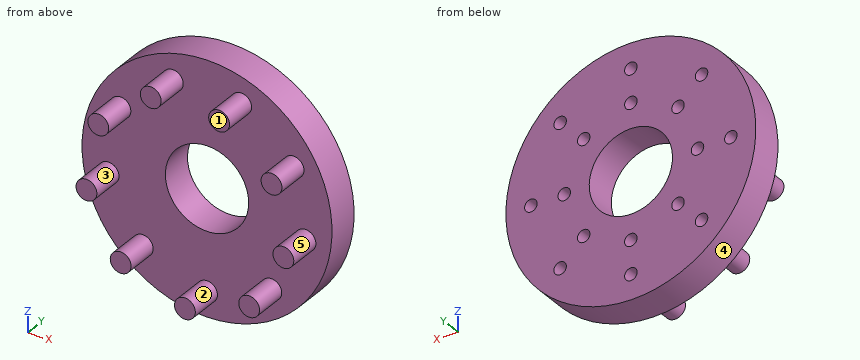
from build123d import *

# Parameters (mm, degrees)
SKETCH1_R           = 190.5
BOSS_EXTRUDE1_DEPTH = 50.8
SKETCH2_R           = 63.5
CUT_EXTRUDE1_DEPTH  = 275.155320941
SKETCH3_R           = 9.525
CUT_EXTRUDE2_DEPTH  = 42.926
SKETCH4_R           = 15.875
BOSS_EXTRUDE2_DEPTH = 50.8


with BuildPart() as part:
    # Sketch1 → Boss-Extrude1 (new body)
    with BuildSketch(Plane(origin=(0, 0, 0), x_dir=(1, 0, 0), z_dir=(0, 1, 0))):
        with Locations(Location((0, 0, 0), (0, 0, 270))):
            Circle(SKETCH1_R)
    extrude(amount=BOSS_EXTRUDE1_DEPTH)

    # Sketch2 → Cut-Extrude1 (cut, through all)
    with BuildSketch(Plane(origin=(0, 50.8, 0), x_dir=(1, 0, 0), z_dir=(0, 1, 0))):
        with Locations(Location((0, 0, 0), (0, 0, 270))):
            Circle(SKETCH2_R)
    extrude(amount=-CUT_EXTRUDE1_DEPTH, mode=Mode.SUBTRACT)

    # Sketch3 → Cut-Extrude2 (cut)
    with BuildSketch(Plane(origin=(0, 50.8, 0), x_dir=(1, 0, 0), z_dir=(0, 1, 0))):
        with Locations(Location((0, 101.6, 0), (0, 0, 270))):
            Circle(SKETCH3_R)
        with Locations(Location((71.842048969, 71.842048969, 0), (0, 0, 270))):
            Circle(SKETCH3_R)
        with Locations(Location((101.6, 0, 0), (0, 0, 270))):
            Circle(SKETCH3_R)
        with Locations(Location((71.842048969, -71.842048969, 0), (0, 0, 270))):
            Circle(SKETCH3_R)
        with Locations(Location((0, -101.6, 0), (0, 0, 270))):
            Circle(SKETCH3_R)
        with Locations(Location((-71.842048969, -71.842048969, 0), (0, 0, 270))):
            Circle(SKETCH3_R)
        with Locations(Location((-101.6, 0, 0), (0, 0, 270))):
            Circle(SKETCH3_R)
        with Locations(Location((-71.842048969, 71.842048969, 0), (0, 0, 270))):
            Circle(SKETCH3_R)
        with Locations(Location((0, 152.4, 0), (0, 0, 270))):
            Circle(SKETCH3_R)
        with Locations(Location((107.763073453, 107.763073453, 0), (0, 0, 270))):
            Circle(SKETCH3_R)
        with Locations(Location((152.4, 0, 0), (0, 0, 270))):
            Circle(SKETCH3_R)
        with Locations(Location((107.763073453, -107.763073453, 0), (0, 0, 270))):
            Circle(SKETCH3_R)
        with Locations(Location((0, -152.4, 0), (0, 0, 270))):
            Circle(SKETCH3_R)
        with Locations(Location((-107.763073453, -107.763073453, 0), (0, 0, 270))):
            Circle(SKETCH3_R)
        with Locations(Location((-152.4, 0, 0), (0, 0, 270))):
            Circle(SKETCH3_R)
        with Locations(Location((-107.763073453, 107.763073453, 0), (0, 0, 270))):
            Circle(SKETCH3_R)
    extrude(amount=-CUT_EXTRUDE2_DEPTH, mode=Mode.SUBTRACT)

    # Sketch4 → Boss-Extrude2 (add)
    with BuildSketch(Plane.XZ):
        with Locations(Location((0, -152.4, 0), (0, 0, 90))):
            Circle(SKETCH4_R)
        with Locations(Location((-97.960831716, -116.745173131, 0), (0, 0, 90))):
            Circle(SKETCH4_R)
        with Locations(Location((-150.084701559, -26.463982276, 0), (0, 0, 90))):
            Circle(SKETCH4_R)
        with Locations(Location((-131.982271537, 76.2, 0), (0, 0, 90))):
            Circle(SKETCH4_R)
        with Locations(Location((-52.123869843, 143.209155408, 0), (0, 0, 90))):
            Circle(SKETCH4_R)
        with Locations(Location((52.123869843, 143.209155408, 0), (0, 0, 90))):
            Circle(SKETCH4_R)
        with Locations(Location((131.982271537, 76.2, 0), (0, 0, 90))):
            Circle(SKETCH4_R)
        with Locations(Location((150.084701559, -26.463982276, 0), (0, 0, 90))):
            Circle(SKETCH4_R)
        with Locations(Location((97.960831716, -116.745173131, 0), (0, 0, 90))):
            Circle(SKETCH4_R)
    extrude(amount=BOSS_EXTRUDE2_DEPTH)


solid = part.part
Model file for the job. Use its own axes, mm. Face numbers are marked on the shaded views. A direction names the side the tool comes from. Coordinates: 2 decimals unless noted, no trailing zeros. Write each loop counter-clockwise with the first axis right and the second up, starting at its lowest first coordinate (ties: lowest second). Pieces come first, ordered by that corner, then holes. Notation, with made-up numbers: (44, 43) - (68, 43) arc R21 ccw to (68, 58) - close; hole circle Ø4 at (-38.5, 0). An arc over 180 degrees is marked (long way). Write each question's results on one line, items separated by ' | '. Start each with the question number.
1) Flat gauge pins, fed straight in: P1, Ø12, axis at x = -56, z = 70, coming from the -Y side; P2, Ø3, axis at x = -59.5, y = -28.5, coming from the +Z side; P3, Ø5.5, axis at x = 104, z = -3.5, coming from the +Y side; P4, Ø12, axis at x = -27, y = -20, coming from the +Z side. Where does each tip first touch, or does it go through?
2) Cut at A-A (x = 0). Write the cut outline in (y, z) (3 decimals).
3) 3-axis set-ups, long thin cutter, end or side, ignore diameter. For the marked faces 4 and 5: which of +Z, -Z, +X, -X, +Y, -Y reach the whole face in a straight line?
4) Mould opens along X. For the marked faces 1, 2 and 3 say: pulls with the +X half, pulls with the -X half, needs draft (parallel to the pull), parting line crosses it, or undercut.
5) Probe line 1 along X through (y, z) = (24.5, 0) (3 decimals); line 2 along X through (y, z) = (27, 71.5); line 3 along X through (y, z) = (41, 69.5). List the from-to ranges inside material, lowest first. Write a range as from..to.
6) Cut at B-B (z = 24.5). Write the cut outline in (x, y).
7) Cut at C-C (y = -31.5). Count the separate pieces of the cut face and the enclosed holes in it, then the cut area to 3 significant figures.
8) Cut at D-D (z = 76.2). Write the cut outline in (x, y).
Returned:
1) P1: y = 0 | P2: z = 157.96 | P3: y = 7.87 | P4: through
2) outline: (-50.8, -168.275) - (0, -168.275) - (0, -190.5) - (50.8, -190.5) - (50.8, -161.925) - (7.874, -161.925) - (7.874, -142.875) - (50.8, -142.875) - (50.8, -111.125) - (7.874, -111.125) - (7.874, -92.075) - (50.8, -92.075) - (50.8, -63.5) - (0, -63.5) - (0, -136.525) - (-50.8, -136.525) - close; (0, 63.5) - (50.8, 63.5) - (50.8, 92.075) - (7.874, 92.075) - (7.874, 111.125) - (50.8, 111.125) - (50.8, 142.875) - (7.874, 142.875) - (7.874, 161.925) - (50.8, 161.925) - (50.8, 190.5) - (0, 190.5) - close
3) face 4: +Y, -Y | face 5: -Y
4) face 1: needs draft | face 2: parting line crosses it | face 3: undercut
5) line 1: -190.5..-161.925, -142.875..-111.125, -92.075..-63.5, 63.5..92.075, 111.125..142.875, 161.925..190.5 | line 2: -176.57..-81.36, -62.32..62.32, 81.36..176.57 | line 3: -177.37..-81.07, -62.61..62.61, 81.07..177.37
6) outline: (-188.92, 0) - (-58.58, 0) - (-58.58, 50.8) - (-188.92, 50.8) - close; (58.58, 0) - (188.92, 0) - (188.92, 50.8) - (58.58, 50.8) - close
7) separate pieces: 9 | enclosed holes: 0 | area: 7,130 mm^2
8) outline: (-174.6, 0) - (-147.86, 0) - (-147.86, -50.8) - (-116.11, -50.8) - (-116.11, 0) - (116.11, 0) - (116.11, -50.8) - (147.86, -50.8) - (147.86, 0) - (174.6, 0) - (174.6, 50.8) - (80.31, 50.8) - (80.31, 7.87) - (63.37, 7.87) - (63.37, 50.8) - (-63.37, 50.8) - (-63.37, 7.87) - (-80.31, 7.87) - (-80.31, 50.8) - (-174.6, 50.8) - close
